Verification items for the finished model (mm, model axes). Give positions to 0.01 mm unless a question says otherwise; leave off trailing zeros. Use CSV: the item, a comma, the result in double quotes.
from build123d import *

# Parameters (mm, degrees)
SKETCH2_R           = 19.05
BOSS_EXTRUDE1_DEPTH = 5.08
SKETCH3_R           = 1
CUT_EXTRUDE1_DEPTH  = 28.415532094
FILLET1_R           = 2.54


with BuildPart() as part:
    # Sketch2 → Boss-Extrude1 (new body)
    with BuildSketch(Plane(origin=(0, 0, 0), x_dir=(1, 0, 0), z_dir=(0, 1, 0))):
        with Locations(Location((0, 0, 0), (0, 0, 270))):
            Circle(SKETCH2_R)
    extrude(amount=BOSS_EXTRUDE1_DEPTH)

    # Sketch3 → Cut-Extrude1 (cut, through all)
    with BuildSketch(Plane(origin=(0, 5.08, 0), x_dir=(1, 0, 0), z_dir=(0, 1, 0))):
        with Locations(Location((-6.75, -11.691342951, 0), (0, 0, 270))):
            Circle(SKETCH3_R)
        with Locations(Location((-5.25, -9.09326674, 0), (0, 0, 270))):
            Circle(SKETCH3_R)
        with Locations(Location((-3.75, -6.495190528, 0), (0, 0, 270))):
            Circle(SKETCH3_R)
        with Locations(Location((-13.5, 0, 0), (0, 0, 270))):
            Circle(SKETCH3_R)
        with Locations(Location((-10.5, 0, 0), (0, 0, 270))):
            Circle(SKETCH3_R)
        with Locations(Location((-7.5, 0, 0), (0, 0, 270))):
            Circle(SKETCH3_R)
        with Locations(Location((-3.75, 6.495190528, 0), (0, 0, 270))):
            Circle(SKETCH3_R)
        with Locations(Location((-5.25, 9.09326674, 0), (0, 0, 270))):
            Circle(SKETCH3_R)
        with Locations(Location((-6.75, 11.691342951, 0), (0, 0, 270))):
            Circle(SKETCH3_R)
        with Locations(Location((6.75, 11.691342951, 0), (0, 0, 270))):
            Circle(SKETCH3_R)
        with Locations(Location((5.25, 9.09326674, 0), (0, 0, 270))):
            Circle(SKETCH3_R)
        with Locations(Location((3.75, 6.495190528, 0), (0, 0, 270))):
            Circle(SKETCH3_R)
        with Locations(Location((13.5, 0, 0), (0, 0, 270))):
            Circle(SKETCH3_R)
        with Locations(Location((10.5, 0, 0), (0, 0, 270))):
            Circle(SKETCH3_R)
        with Locations(Location((7.5, 0, 0), (0, 0, 270))):
            Circle(SKETCH3_R)
        with Locations(Location((3.75, -6.495190528, 0), (0, 0, 270))):
            Circle(SKETCH3_R)
        with Locations(Location((5.25, -9.09326674, 0), (0, 0, 270))):
            Circle(SKETCH3_R)
        with Locations(Location((6.75, -11.691342951, 0), (0, 0, 270))):
            Circle(SKETCH3_R)
    extrude(amount=-CUT_EXTRUDE1_DEPTH, mode=Mode.SUBTRACT)

    # Fillet1
    fillet1_edges = [part.edges().sort_by_distance(p)[0] for p in [
        (0, 0, -19.05),
        (0, 5.08, -19.05),
    ]]
    fillet(fillet1_edges, radius=FILLET1_R - 0.0001)  # a hair under: the kernel refuses the full size


solid = part.part
(1) Mould release check, pull along Z, two halves, no side actions. Record for faces 1 (the flat face through (0, 0, 0)), 2 (the cylindrical face through (-14.476, 2.576, -0.217)): released by +Z, released by -Z, zero draft, split by the parting line, or undercut.
Calculated:
face 1,"zero draft"
face 2,"undercut"
(2) Scan lines: L1, parallel to X at y = 4.3, z = 8.5 (3 decimals); L2, parallel to Z at x = -4.5, y = 0.95; L3, parallel to X at y = 3.25, z = 12.5. Record each from-to range of solid material in increasing order. Write a range as from..to.
Calculated:
L1,"x = -16.253..-6.055, -4.445..4.445, 6.055..16.253"
L2,"z = -17.93..-9.75, -8.43..-7.16, -5.83..5.83, 7.16..8.43, 9.75..17.93"
L3,"x = -14.24..-7.34, -6.16..6.16, 7.34..14.24"
(3) Depth check by flat-ended pin: pin 1 Ø2.5 at (x, z) = (10.5, 0) entering from +Y; pin 2 Ø1.5 at (x, y) = (13.5, 1.5) entering from -Z. Enter the tip coordinate at first touch or a pass-through.
Calculated:
pin 1,"stops at y = 5.08"
pin 2,"stops at z = -13.95"
(4) Section check A-A on y = 3.2. Count the separate pieces of the cut face and the enclosed holes in it, plus the area to 3 significant figures.
Calculated:
separate pieces,"1"
enclosed holes,"18"
area,"1,070 mm²"
